Input: part model. Units: mm. Frame: model coordinates. Coordinates: 2 decimals unless noted, no trailing zeros.
Item 1: Contact query for flat-ended pins moving along their axis: P1, Ø3, axis at x = 6, z = 183.5, coming from the +Y side; P2, Ø3, axis at x = 6, z = 260, coming from the -Y side. Output: stop coordinate, or through.
Item 2: Ray query, line 1 along X through (y, z) = (2.4, 235); line 2 along X through (y, z) = (5.6, 210); line 3 along Y through (x, z) = (3.75, 333.5). Return the intervals inside material, ascending.
Item 3: Section A-A on y = 3.75. Give the number of separate pieces and of enclosed holes in the cut face, and give its area (3 significant figures).
```python
from build123d import *

# Parameters (mm, degrees)
SKETCH1_W                      = 12
SKETCH1_H                      = 8
BOSS_EXTRUDE1_DEPTH            = 395
CBORE_FOR_M3_SHCS1_D           = 3.4
CBORE_FOR_M3_SHCS1_CBORE_D     = 6.5
CBORE_FOR_M3_SHCS1_CBORE_DEPTH = 3


with BuildPart() as part:
    # Sketch1 → Boss-Extrude1 (new body)
    with BuildSketch(Plane.XY):
        with Locations((6, 4)):
            Rectangle(SKETCH1_W, SKETCH1_H)
    extrude(amount=BOSS_EXTRUDE1_DEPTH)

    # CBORE for M3 SHCS1 (through all)
    with Locations(Plane(origin=(0, 8, 0), x_dir=(1, 0, 0), z_dir=(0, 1, 0))):
        with Locations((6, -385), (6, -360), (6, -335), (6, -310), (6, -285), (6, -260), (6, -235), (6, -210), (6, -185), (6, -160), (6, -135), (6, -110), (6, -85), (6, -60), (6, -35), (6, -10)):
            CounterBoreHole(CBORE_FOR_M3_SHCS1_D / 2, CBORE_FOR_M3_SHCS1_CBORE_D / 2, CBORE_FOR_M3_SHCS1_CBORE_DEPTH)


solid = part.part
```
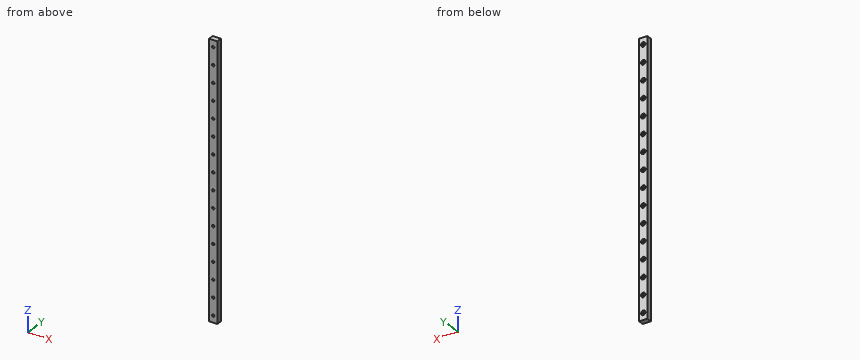
Results found:
1. P1: stops at y = 5
1. P2: passes through
2. line 1: x = 0 to 4.3, 7.7 to 12
2. line 2: x = 0 to 2.75, 9.25 to 12
2. line 3: y = 0 to 5
3. separate pieces: 1
3. enclosed holes: 16
3. area: 4,590 mm2
